Part model, mm, in its own coordinate system. Round coordinates to 2 decimals unless told otherwise and drop trailing zeros. Write each loop counter-clockwise with the first axis right and the second up, starting at its lowest first coordinate (ties: lowest second). Pieces come first, ordered by that corner, then holes. Notation, with made-up numbers: (61, 74) -> (117, 74) arc R30 cw to (117, 100) -> close; hole circle Ø7 at (41.25, -33). An arc over 180 degrees is marked (long way). Use CSV: the item, a comma, the result in double quotes. Start each with the question number.
(1) Probe line 1 (X direction, y = -889.5, z = 72.5); line 2 (X direction, y = -736, z = 80). List the from-to ranges inside material, lowest first. Write a range as [from, to].
(2) Saw through at A-A (z = -2.5). Give the cut face in (x, y), plus the area to 3 significant figures.
(3) Drop a flat-ended pin along its axis: pin 1 (1.5 mm diameter, centred on y = -593.5, z = 58, fed in from -X). Give the stop position or say it passes through.
```python
from build123d import *

# Parameters (mm, degrees)
F1_DEPTH = 25.4
F2_DEPTH = 508
F3_DEPTH = 508
F4_DEPTH = 508


with BuildPart() as f1:
    # F0 (on Front) → F1 (new body)
    with BuildSketch(Plane.XZ):
        Polygon((86.5744352341, 88.8054594398), (-86.4560827613, 88.8054594398), (-77.5985121727, -82.9327851534), (86.5744352341, -82.9327851534), align=None)
    extrude(amount=F1_DEPTH)

    # F2 (add): a face of the model
    f2_faces = [f1.faces().sort_by_distance(p)[0] for p in [
        (2.2541798586, -25.4, 3.688199535),
    ]]
    extrude(f2_faces, amount=F2_DEPTH)

    # F3 (add): a face of the model
    f3_faces = [f1.faces().sort_by_distance(p)[0] for p in [
        (2.2541798586, -533.4, 3.688199535),
    ]]
    extrude(f3_faces, amount=F3_DEPTH)

    # F4 (add): a face of the model
    f4_faces = [f1.faces().sort_by_distance(p)[0] for p in [
        (0.0591762364, -520.7, 88.8054594398),
    ]]
    extrude(f4_faces, amount=F4_DEPTH)


solid = f1.part
```
Answers:
1,line 1,"x = [-85.62, 86.57]"
1,line 2,"x = [-86, 86.57]"
2,outline,"(-81.75, -1041.4) -> (86.57, -1041.4) -> (86.57, 0) -> (-81.75, 0) -> close"
2,area,"175,000 mm²"
3,pin 1,"stops at x = -84.91"
